Source: CAD feature listing. Evaluate the final solid. Frame: model axes, mm. A direction names the side the tool comes from. Round coordinates to 2 decimals unless told otherwise and drop trailing zeros. Order: outer loops, then holes, each group sorted by start corner. A loop starts at its lowest first (then second) coordinate and runs counter-clockwise, first axis right, second up. Notation, with made-up numbers: (47, -16.5) - (103, -16.5) arc R17 ccw to (103, 7.5) - close; hole circle Ø5 at (45.5, -39.5). An arc over 180 degrees is marked (long way). Put each result on its own line as item: value. Start each with the question number.
1) Section D-D on x = -2.25. Output: boundary loops of the cut face in (y, z) (1 decimal), then the cut area to 3 significant figures.
2) Contact query for flat-ended pins moving along their axis: P1, Ø1, axis at y = 40, z = 0, coming from the +X side; P2, Ø1, axis at x = 1.5, z = 0, coming from the -Y side (3 decimals); P3, Ø1.5, axis at y = 54, z = 0.5, coming from the -X side. Output: stop coordinate, or through.
3) Mould query, pull axis Y, two halves, no side actions, for faces 4 (the face through (-10, 63.35, 0)), 5 (the face through (-10, 7.175, 0)), 6 (the face through (3.175, 18, 0)), 7 (the face through (-22, 14.675, 0)). Classes: +Y half, -Y half, draft (parallel to the pull), parting line (faces both ways), or undercut.
4) Line query: probe 1 along Y at (x, z) = (-21.25, 0) (3 decimals); probe 2 along Y at (x, z) = (-11.5, 1.25) (3 decimals); probe 3 along X at (y, z) = (39.5, -1.2). Output: solid intervals per line, ascending. Write a range as [from, to].
5) Section A-A on y = 6.5. Output: boundary loops of the cut face in (x, z), then the cut area to 3 significant figures.
6) Section B-B on x = 1.75. Output: boundary loops of the cut face in (y, z) (1 decimal), then the cut area to 4 significant figures.
7) Access query for faces 1 (the face through (0, 56, 0)), 2 (the face through (2, 20.675, 0)), 3 (the face through (-20, 56, 0)). Directions: +Z, -Z, +X, -X, +Y, -Y. A direction counts if a zero-diameter tool reaches every point of the face in a straight line with its end or side. Return the directions, or none.
```python
from build123d import *

# Parameters (mm, degrees)
SKETCH1_W           = 9
SKETCH1_H           = 3.175
BOSS_EXTRUDE2_DEPTH = 1.5875


with BuildPart() as part:
    # Sketch1 → Boss-Extrude2 (new body, symmetric)
    with BuildSketch(Plane.XY):
        Polygon((0, 14.675), (3.175, 14.675), (3.175, 20.675), (0, 20.675), (0, 30.675), (3.175, 30.675), (3.175, 36.675), (0, 36.675), (0, 46.675), (3.175, 46.675), (3.175, 52.675), (0, 52.675), (0, 60.175), (-5.5, 60.175), (-5.5, 63.35), (-14.5, 63.35), (-14.5, 60.175), (-20, 60.175), (-20, 52.675), (-23.175, 52.675), (-23.175, 46.675), (-20, 46.675), (-20, 36.675), (-23.175, 36.675), (-23.175, 30.675), (-20, 30.675), (-20, 20.675), (-23.175, 20.675), (-23.175, 14.675), (-20, 14.675), (-20, 7.175), (-20, 0), (0, 0), (0, 7.175), align=None)
        with Locations((-10, 5.5875)):
            Rectangle(SKETCH1_W, SKETCH1_H, mode=Mode.SUBTRACT)
    extrude(amount=BOSS_EXTRUDE2_DEPTH, both=True)


solid = part.part
```
Answer sheet:
1. outline: (0, -1.6) - (60.2, -1.6) - (60.2, 1.6) - (0, 1.6) - close
1. area: 191 mm^2
2. P1: x = 0
2. P2: y = 14.675
2. P3: x = -20
3. face 4: +Y half
3. face 5: undercut
3. face 6: draft
3. face 7: -Y half
4. probe 1: [14.675, 20.675], [30.675, 36.675], [46.675, 52.675]
4. probe 2: [0, 4], [7.175, 63.35]
4. probe 3: [-20, 0]
5. outline: (-20, -1.59) - (-14.5, -1.59) - (-14.5, 1.59) - (-20, 1.59) - close; (-5.5, -1.59) - (0, -1.59) - (0, 1.59) - (-5.5, 1.59) - close
5. area: 34.9 mm^2
6. outline: (14.7, -1.6) - (20.7, -1.6) - (20.7, 1.6) - (14.7, 1.6) - close; (30.7, -1.6) - (36.7, -1.6) - (36.7, 1.6) - (30.7, 1.6) - close; (46.7, -1.6) - (52.7, -1.6) - (52.7, 1.6) - (46.7, 1.6) - close
6. area: 57.15 mm^2
7. face 1: +Z, -Z, +X, +Y
7. face 2: +Z, -Z, +X
7. face 3: +Z, -Z, -X, +Y
